Read the model definition and answer for the solid it produces. Units are mm, in the model's axes. A direction names the side the tool comes from. Round coordinates to 2 decimals unless told otherwise and drop trailing zeros. Write each loop counter-clockwise with the first axis right and the second up, starting at its lowest first coordinate (ties: lowest second). Pieces come first, ordered by that corner, then holes. Notation, with made-up numbers: (65, 67) -> (97, 67) arc R27 ccw to (97, 85) -> close; hole circle Ø4 at (13, 85). An arc over 180 degrees is marked (long way). Return JSON: item names as keys, results as strings. Group by question number.
(1) A cutting plane is placed at D-D on z = 0.7. Give the vertices of the cut face in (x, y), then the cut area to 3 significant figures.
(2) Straight lines are drawn through the part: line 1 (Y direction, x = 5.5, z = 2.8); line 2 (Y direction, x = -8.5, z = 1.7); line 3 (X direction, y = -1.25, z = 2.6). For each, find the intervals that lie inside material, in ascending order.
(3) A cutting plane is placed at C-C on y = -5.75. Give the vertices of the cut face in (x, z), then the cut area to 3 significant figures.
(4) A cutting plane is placed at A-A on x = 9. Give the vertices of the cut face in (y, z).
(5) A cutting plane is placed at B-B on z = 2.9. Give the vertices of the cut face in (x, y).
(6) The mould has two halves that part along Y. Classify faces 1 (the flat face through (3, -16, 2)), 2 (the flat face through (-6, 2.5, 2)), 3 (the flat face through (-13, -14, 2.4)): released by +Y, released by -Y, zero draft, split by the parting line, or undercut.
(7) For faces 4 (the flat face through (3, 1, 2)), 5 (the flat face through (-3, -14.7, 2)), 6 (the flat face through (1, -2.5, 2)), 7 (the flat face through (9, -15.9, 2)), determine the directions among +Z, -Z, +X, -X, +Y, -Y from which every point of the face is accessible in a straight line to the end or side of a thin tool.
(8) Given pin 1 (0.5 mm diameter, centred on x = 9, z = 2, fed in from -Y); pin 2 (1 mm diameter, centred on x = -8, z = 2, fed in from +Y); pin 3 (0.8 mm diameter, centred on x = 3.5, z = 1, fed in from +Y), each flat-ended and moving along its own axis, determine where each tip first touches the part or whether it passes through.
```python
from build123d import *

# Parameters (mm, degrees)
F0_W        = 21.3
F0_H        = 2.5
F0_R        = 1.55
F1_DEPTH    = 3.4
F0_W_2      = 1.2
F0_H_2      = 1.2
F0_W_3      = 3.5
F2_DEPTH    = 3.4
F0_H_3      = 12.2
F3_DEPTH    = 1.2
F4_W        = 5
F4_H        = 1
F5_DEPTH    = 2
F6_T4_DEPTH = 3.4
F6_T9_DEPTH = 3.4


# Not quite as in the source:
# - a fillet or chamfer that OpenCascade refuses, or shapes differently, is made with other operations: its cross-section is extruded or revolved along the edge and cut away or added
# - a feature names something its author has since deleted; it is built from what else it names


with BuildPart() as f1:
    # F0 (on Top) → F1 (new body)
    with BuildSketch(Plane.XY):
        with BuildLine():
            ThreePointArc((-16.4319353276, -0.9810708435), (-15.752751994, 1.4598801321), (-13.6819353276, 0))
            ThreePointArc((-13.6819353276, 0), (-14.1359198167, -1.0960155108), (-15.2319353276, -1.55))
            Line((-15.2319353276, -1.55), (-15.2319353276, -2.5))
            Line((-15.2319353276, -2.5), (-13.1552793618, -2.5))
            ThreePointArc((-13.1552793618, -2.5), (-12.2898585195, -1.3808273084), (-11.9819353276, 0))
            ThreePointArc((-11.9819353276, 0), (-12.2898585195, 1.3808273084), (-13.1552793618, 2.5))
            ThreePointArc((-13.1552793618, 2.5), (-18.0266966766, 1.6588577401), (-16.4319353276, -3.0203476621))
            Line((-16.4319353276, -3.0203476621), (-16.4319353276, -2.5))
            Line((-16.4319353276, -2.5), (-16.4319353276, -0.9810708435))
        make_face()
        with BuildLine():
            ThreePointArc((-15.2319353276, -1.55), (-15.8959534721, -1.4005641377), (-16.4319353276, -0.9810708435))
            Line((-16.4319353276, -0.9810708435), (-16.4319353276, -2.5))
            Line((-16.4319353276, -2.5), (-15.2319353276, -2.5))
            Line((-15.2319353276, -2.5), (-15.2319353276, -1.55))
        make_face()
        with BuildLine():
            ThreePointArc((-11.9819353276, 0), (-12.2898585195, -1.3808273084), (-13.1552793618, -2.5))
            Line((-13.1552793618, -2.5), (-11.7319353276, -2.5))
            Line((-11.7319353276, -2.5), (-11.7319353276, 0))
            Line((-11.7319353276, 0), (-11.9819353276, 0))
        make_face()
        with BuildLine():
            Line((1.7680646724, 2.5), (-13.1552793618, 2.5))
            ThreePointArc((-13.1552793618, 2.5), (-12.2898585195, 1.3808273084), (-11.9819353276, 0))
            Line((-11.9819353276, 0), (-11.7319353276, 0))
            Line((-11.7319353276, 0), (9.5680646724, 0))
            Line((9.5680646724, 0), (9.5680646724, -2.5))
            Line((9.5680646724, -2.5), (13.4914087067, -2.5))
            ThreePointArc((13.4914087067, -2.5), (12.3180646724, 0), (13.4914087067, 2.5))
            Line((13.4914087067, 2.5), (4.5180646724, 2.5))
            Line((4.5180646724, 2.5), (4.5180646724, 1))
            Line((4.5180646724, 1), (1.7680646724, 1))
            Line((1.7680646724, 1), (1.7680646724, 2.5))
        make_face()
        with Locations((-1.0819353276, -1.25)):
            Rectangle(F0_W, F0_H)
        with BuildLine():
            ThreePointArc((13.4914087067, 2.5), (12.3180646724, 0), (13.4914087067, -2.5))
            Line((13.4914087067, -2.5), (17.6447206382, -2.5))
            ThreePointArc((17.6447206382, -2.5), (18.5101414805, -1.3808273084), (18.8180646724, 0))
            ThreePointArc((18.8180646724, 0), (16.9488919809, 2.942076808), (13.4914087067, 2.5))
        make_face()
        with Locations((15.5680646724, 0)):
            Circle(F0_R, mode=Mode.SUBTRACT)
    extrude(amount=F1_DEPTH)

    # F0 (on Top) → F2 (join)
    with BuildSketch(Plane.XY):
        with BuildLine():
            ThreePointArc((-15.2319353276, -3.25), (-15.8428240646, -3.1920706369), (-16.4319353276, -3.0203476621))
            Line((-16.4319353276, -3.0203476621), (-16.4319353276, -14.7))
            Line((-16.4319353276, -14.7), (-15.2319353276, -14.7))
            Line((-15.2319353276, -14.7), (-15.2319353276, -3.25))
        make_face()
        with BuildLine():
            Line((-15.2319353276, -2.5), (-16.4319353276, -2.5))
            Line((-16.4319353276, -2.5), (-16.4319353276, -3.0203476621))
            ThreePointArc((-16.4319353276, -3.0203476621), (-15.8428240646, -3.1920706369), (-15.2319353276, -3.25))
            Line((-15.2319353276, -3.25), (-15.2319353276, -2.5))
        make_face()
        with Locations((-15.8319353276, -15.3)):
            Rectangle(F0_W_2, F0_H_2)
        with Locations((-13.4819353276, -15.3)):
            Rectangle(F0_W_3, F0_H_2)
        Polygon((9.5680646724, -14.7), (-11.7319353276, -14.7), (-11.7319353276, -15.9), (-0.2319353276, -15.9), (7.0180646724, -15.9), (9.5680646724, -15.9), align=None)
        Polygon((7.0180646724, -15.9), (-0.2319353276, -15.9), (-0.2319353276, -16.7), (1.7680646724, -16.7), (1.7680646724, -16), (4.5180646724, -16), (4.5180646724, -16.7), (7.0180646724, -16.7), align=None)
    extrude(amount=F2_DEPTH)

    # F0 (on Top) → F3 (join)
    with BuildSketch(Plane.XY):
        with BuildLine():
            ThreePointArc((-13.1552793618, -2.5), (-14.1279652193, -3.0567548152), (-15.2319353276, -3.25))
            Line((-15.2319353276, -3.25), (-15.2319353276, -14.7))
            Line((-15.2319353276, -14.7), (-11.7319353276, -14.7))
            Line((-11.7319353276, -14.7), (-11.7319353276, -2.5))
            Line((-11.7319353276, -2.5), (-13.1552793618, -2.5))
        make_face()
        with BuildLine():
            Line((-13.1552793618, -2.5), (-15.2319353276, -2.5))
            Line((-15.2319353276, -2.5), (-15.2319353276, -3.25))
            ThreePointArc((-15.2319353276, -3.25), (-14.1279652193, -3.0567548152), (-13.1552793618, -2.5))
        make_face()
        with Locations((-1.0819353276, -8.6)):
            Rectangle(F0_W, F0_H_3)
    extrude(amount=F3_DEPTH)

    # F4 (on face) → F5 (join)
    with BuildSketch(Plane(origin=(0, -14.7, 0), x_dir=(-1, 0, 0), z_dir=(0, 1, 0))):
        with Locations((12.7319353276, 2.9)):
            Rectangle(F4_W, F4_H)
    extrude(amount=F5_DEPTH)

    # F6: chamfer of 1.5 on 2 edges, made by hand


with BuildPart() as f6_tool2:
    # F6_s3 → F6_t4 (new body)
    with BuildSketch(Plane.XY):
        Polygon((-1.7319353276, -15.9), (-0.2319353276, -17.4), (-0.2319353276, -15.9), align=None)
    extrude(amount=F6_T4_DEPTH)

    split(bisect_by=Plane.XZ.offset(16.7), keep=Keep.BOTTOM)


with BuildPart() as f1_1:
    add(f1.part)

    # F6_t1: union F6_tool2
    add(f6_tool2.part)


with BuildPart() as f6_tool7:
    # F6_s8 → F6_t9 (new body)
    with BuildSketch(Plane.XY):
        Polygon((7.0180646724, -17.4), (8.5180646724, -15.9), (7.0180646724, -15.9), align=None)
    extrude(amount=F6_T9_DEPTH)

    split(bisect_by=Plane.XZ.offset(16.7), keep=Keep.BOTTOM)


with BuildPart() as f1_2:
    add(f1_1.part)

    # F6_t6: union F6_tool7
    add(f6_tool7.part)


solid = f1_2.part
```
Checks:
{
 "1": {"outline": "(-16.43, -15.9) -> (-1.73, -15.9) -> (-0.93, -16.7) -> (1.77, -16.7) -> (1.77, -16) -> (4.52, -16) -> (4.52, -16.7) -> (7.72, -16.7) -> (8.52, -15.9) -> (9.57, -15.9) -> (9.57, -2.5) -> (17.64, -2.5) arc R3.25 ccw to (13.49, 2.5) -> (4.52, 2.5) -> (4.52, 1) -> (1.77, 1) -> (1.77, 2.5) -> (-13.16, 2.5) arc R3.25 ccw (long way) to (-16.43, -3.02) -> close; hole circle Ø3.1 at (-15.23, 0); hole circle Ø3.1 at (15.57, 0)", "area": "522 mm^2"},
 "2": {"line 1": "y = -16.7 to -14.7, -2.5 to 2.5", "line 2": "y = -15.9 to -14.7, -2.5 to 2.5", "line 3": "x = -18.23 to -16.15, -14.32 to 14.65, 16.48 to 18.57"},
 "3": {"outline": "(-16.43, 0) -> (9.57, 0) -> (9.57, 1.2) -> (-15.23, 1.2) -> (-15.23, 3.4) -> (-16.43, 3.4) -> close", "area": "33.8 mm^2"},
 "4": {"outline": "(-15.9, 0) -> (2.5, 0) -> (2.5, 3.4) -> (-2.5, 3.4) -> (-2.5, 1.2) -> (-14.7, 1.2) -> (-14.7, 3.4) -> (-15.9, 3.4) -> close"},
 "5": {"outline": "(-16.43, -15.9) -> (-1.73, -15.9) -> (-0.93, -16.7) -> (1.77, -16.7) -> (1.77, -16) -> (4.52, -16) -> (4.52, -16.7) -> (7.72, -16.7) -> (8.52, -15.9) -> (9.57, -15.9) -> (9.57, -14.7) -> (-10.23, -14.7) -> (-10.23, -12.7) -> (-15.23, -12.7) -> (-15.23, -2.5) -> (17.64, -2.5) arc R3.25 ccw to (13.49, 2.5) -> (4.52, 2.5) -> (4.52, 1) -> (1.77, 1) -> (1.77, 2.5) -> (-13.16, 2.5) arc R3.25 ccw (long way) to (-16.43, -3.02) -> close; hole circle Ø3.1 at (-15.23, 0); hole circle Ø3.1 at (15.57, 0)"},
 "6": {"face 1": "released by -Y", "face 2": "released by +Y", "face 3": "undercut"},
 "7": {"face 4": "+Z, -Z, +Y", "face 5": "+X", "face 6": "+Z, +X", "face 7": "+Z, -Z, +X, -Y"},
 "8": {"pin 1": "stops at y = -15.9", "pin 2": "stops at y = 2.5", "pin 3": "stops at y = 1"}
}
